Autodesk Fusion 360 part; units mm, degrees
sketch "Sketch1" plane through (0, 0, 0) normal (1, 0, 0) x (0, 0, -1)
  line L0 (0, 0) -> (19, 0)
  line L1 (19, 0) -> (19, 60)
  line L2 (19, 60) -> (0, 60)
  line L3 (0, 60) -> (0, 0)
  circle A0 centre (9.5, 52.5) radius 1.65
  circle A1 centre (9.5, 7.5) radius 1.65
  circle A2 centre (9.5, 30) radius 2.1
  point P0 (9.5, 60)
  point P1 (0, 30)
  dimension "d1" = 3.3
  dimension "d2" = 45
  dimension "d3" = 60
  dimension "d4" = 19
  dimension "d5" = 9.5
  dimension "d6" = 7.5
  dimension "d7" = 4.2
extrude "Extrude1" add sketch "Sketch1" along normal blind 4
sketch "Sketch2" plane through (4, 0, 0) normal (1, 0, 0) x (0, 0, -1)
  circle A0 centre (9.5, 7.5) radius 1.65
  circle A1 centre (9.5, 52.5) radius 1.65
  circle A2 centre (9.5, 30) radius 2.1
  line L0 (0, 60) -> (0, 0)
  line L1 (0, 0) -> (19, 0)
  line L2 (19, 0) -> (19, 60)
  line L3 (19, 60) -> (0, 60)
  line L4 (19, 40.5) -> (0, 40.5)
  line L5 (0, 40.5) -> (0, 19.5)
  line L6 (0, 19.5) -> (19, 19.5)
  line L7 (19, 19.5) -> (19, 40.5)
  line L8 (19, 40.5) -> (0, 19.5) construction
  line L9 (0, 40.5) -> (19, 19.5) construction
  point P0 (9.5, 30)
  dimension "d10" = 21
extrude "Extrude2" cut sketch "Sketch2" against normal blind 1 contours L0 L2 L4 L5 L6 L7
fillet "Fillet1" radius 3 4 edges at (2, 60, 0) (2, 60, -19) (2, 0, -19) (2, 0, 0)
sketch "Sketch3" plane through (0, 0, 0) normal (-1, 0, 0) x (0, 0, 1)
  arc A0 (-3, 0) -> (0, 3) centre (-3, 3) ccw
  line L0 (0, 3) -> (0, 57)
  arc A1 (0, 57) -> (-3, 60) centre (-3, 57) ccw
  line L1 (-3, 60) -> (-16, 60)
  arc A2 (-16, 60) -> (-19, 57) centre (-16, 57) ccw
  line L2 (-19, 57) -> (-19, 3)
  arc A3 (-19, 3) -> (-16, 0) centre (-16, 3) ccw
  line L3 (-16, 0) -> (-3, 0)
  circle A4 centre (-9.5, 7.5) radius 1.65
  circle A5 centre (-9.5, 52.5) radius 1.65
  circle A6 centre (-9.5, 30) radius 2.1
  line L4 (-11.2321, 55.5) -> (-12.9641, 52.5)
  line L5 (-12.9641, 52.5) -> (-11.2321, 49.5)
  line L6 (-11.2321, 49.5) -> (-7.7679, 49.5)
  line L7 (-7.7679, 49.5) -> (-6.0359, 52.5)
  line L8 (-6.0359, 52.5) -> (-7.7679, 55.5)
  line L9 (-7.7679, 55.5) -> (-11.2321, 55.5)
  line L10 (-11.2321, 10.5) -> (-12.9641, 7.5)
  line L11 (-12.9641, 7.5) -> (-11.2321, 4.5)
  line L12 (-11.2321, 4.5) -> (-7.7679, 4.5)
  line L13 (-7.7679, 4.5) -> (-6.0359, 7.5)
  line L14 (-6.0359, 7.5) -> (-7.7679, 10.5)
  line L15 (-7.7679, 10.5) -> (-11.2321, 10.5)
  point P0 (-9.5, 52.5)
  point P1 (-9.5, 7.5)
  dimension "d15" = 6
  dimension "d16" = 6
extrude "Extrude3" cut sketch "Sketch3" against normal blind 3 contours L4 L5 L6 L7 L8 L9 | L10 L11 L12 L13 L14 L15
equation "d5 = d4 / 2"
equation "d16 = d15"
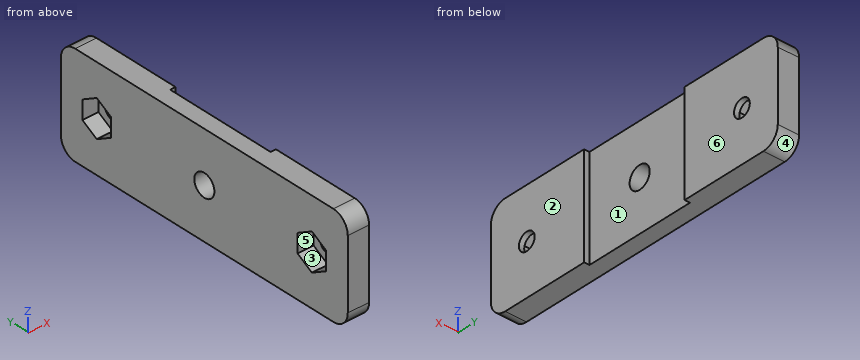
Work out the finished part from the listing and answer in its coordinate system (mm). Face numbers are marked on the shaded views. A direction names the side the tool comes from. Give positions to 0.01 mm unless a question says otherwise; leave off trailing zeros. Order: outer loops, then holes, each group sorted by start corner. A loop starts at its lowest first (then second) coordinate and runs counter-clockwise, first axis right, second up.
1. The mould has two halves that part along Y. Classify the marked faces 4, 5 and 6: released by +Y, released by -Y, zero draft, split by the parting line, or undercut.
Result sheet:
face 4: released by +Y
face 5: undercut
face 6: zero draft
2. Straight lines are drawn through the part: L1, parallel to Y at x = 3.2, z = -9.5; L2, parallel to Y at x = 2.3, z = -9.5; L3, parallel to Z at x = 3.7, y = 7.5. For each, find the intervals that lie inside material, in ascending order.
Result sheet:
L1: y = 0 to 5.85, 9.15 to 19.5, 40.5 to 50.85, 54.15 to 60
L2: y = 0 to 4.5, 10.5 to 27.9, 32.1 to 49.5, 55.5 to 60
L3: z = -19 to -11.15, -7.85 to 0
3. Section B-B, the plane x = 1.1 is taken. Determine the outline of the cut face in (y, z).
Result sheet:
outline: (0, -16) arc R3 ccw to (3, -19) - (57, -19) arc R3 ccw to (60, -16) - (60, -3) arc R3 ccw to (57, 0) - (3, 0) arc R3 ccw to (0, -3) - close; hole (4.5, -11.23) - (7.5, -12.96) - (10.5, -11.23) - (10.5, -7.77) - (7.5, -6.04) - (4.5, -7.77) - close; hole circle Ø4.2 at (30, -9.5); hole (49.5, -11.23) - (52.5, -12.96) - (55.5, -11.23) - (55.5, -7.77) - (52.5, -6.04) - (49.5, -7.77) - close
4. Section A-A, the plane z = -9.5 is taken. Determine the outline of the cut face in (x, y).
Result sheet:
outline: (0, 0) - (4, 0) - (4, 5.85) - (3, 5.85) - (3, 4.5) - (0, 4.5) - close; (0, 10.5) - (3, 10.5) - (3, 9.15) - (4, 9.15) - (4, 19.5) - (3, 19.5) - (3, 27.9) - (0, 27.9) - close; (0, 32.1) - (3, 32.1) - (3, 40.5) - (4, 40.5) - (4, 50.85) - (3, 50.85) - (3, 49.5) - (0, 49.5) - close; (0, 55.5) - (3, 55.5) - (3, 54.15) - (4, 54.15) - (4, 60) - (0, 60) - close
5. Section C-C, the plane y = 29 is taken. Determine the outline of the cut face in (x, z).
Result sheet:
outline: (0, -19) - (3, -19) - (3, -11.35) - (0, -11.35) - close; (0, -7.65) - (3, -7.65) - (3, 0) - (0, 0) - close
6. Section D-D, the plane z = -13.5 is taken. Determine the outline of the cut face in (x, y), and give its area (3 significant figures).
Result sheet:
outline: (0, 0) - (4, 0) - (4, 19.5) - (3, 19.5) - (3, 40.5) - (4, 40.5) - (4, 60) - (0, 60) - close
area: 219 mm2
7. For the marked faces 1, 2 and 3, determine the directions among +Z, -Z, +X, -X, +Y, -Y from which every point of the face is accessible in a straight line to the end or side of a thin tool.
Result sheet:
face 1: +Z, -Z, +X
face 2: +Z, -Z, +X, +Y, -Y
face 3: -X
8. Each of these flat-tipped pins is pushed along its axis until it touches: P1, Ø1.8, axis at y = 52.5, z = -9.5, coming from the -X side; P2, Ø5, axis at y = 7.5, z = -10, coming from the -X side. Where does it stop, or does it pass through?
Result sheet:
P1: passes through
P2: stops at x = 3
